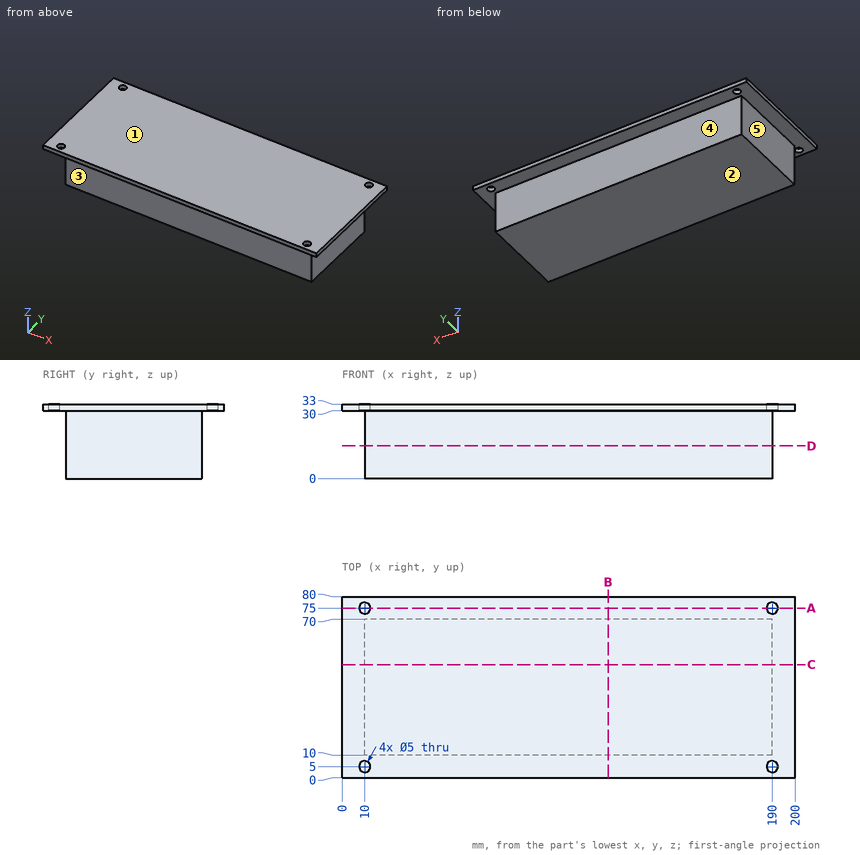
Could you check a few things on this drawing? It's one solid part, dimensions in mm from its lowest x, y, z. A direction names the side the tool comes from. Coordinates: 2 decimals unless noted, no trailing zeros. Order: outer loops, then holes, each group sorted by start corner. A loop starts at its lowest first (then second) coordinate and runs counter-clockwise, first axis right, second up. Notation, with made-up numbers: (11.25, 20.5) -> (56.25, 20.5) arc R17 cw to (56.25, 36.5) -> close; hole circle Ø2 at (-5.75, 52). An arc over 180 degrees is marked (long way). Answer in a Markdown table with one row per item.
(1) I want a section at D-D on z = 14.5. List the corners of the cut face in (x, y) for me, then the cut area to 3 significant figures.
Answer key:
| item | result |
|---|---|
| outline | (10, 10) -> (190, 10) -> (190, 70) -> (10, 70) -> close |
| area | 10,800 mm^2 |
(2) On a 3-axis mill with a long thin cutter (end or side, diameter ignored), from which of +Z, -Z, +X, -X, +Y, -Y can I reach the whole of each face in a straight line? I mean the marked faces 1, 2, 3, 4 and 5. Say none if no direction works.
Answer key:
| item | result |
|---|---|
| face 1 | +Z, +X, -X, +Y, -Y |
| face 2 | -Z, +X, -X, +Y, -Y |
| face 3 | -Z, +X, -X, -Y |
| face 4 | -Z, +X, -X, +Y |
| face 5 | -Z, -X, +Y, -Y |
(3) Will these pins go through, and if not, where does the flat tip stop? pin 1 Ø12 at (y, z) = (14, 22) entering from -X; pin 2 Ø6 at (y, z) = (66.5, 7.5) entering from +X; pin 3 Ø1.5 at (x, z) = (157.5, 23.5) entering from -Y.
Answer key:
| item | result |
|---|---|
| pin 1 | x = 10 |
| pin 2 | x = 190 |
| pin 3 | y = 10 |
(4) I want a section at A-A on y = 75. List the corners of the cut face in (x, z) for me, then the cut area to 3 significant figures.
Answer key:
| item | result |
|---|---|
| outline | (0, 30) -> (7.5, 30) -> (7.5, 33) -> (0, 33) -> close; (12.5, 30) -> (187.5, 30) -> (187.5, 33) -> (12.5, 33) -> close; (192.5, 30) -> (200, 30) -> (200, 33) -> (192.5, 33) -> close |
| area | 570 mm^2 |
(5) Please list where these lines run through material, in increasing order: probe 1 along Y at (x, z) = (10, 31); probe 2 along X at (y, z) = (28, 22); probe 3 along Y at (x, z) = (150, 16).
Answer key:
| item | result |
|---|---|
| probe 1 | 0 to 2.5, 7.5 to 72.5, 77.5 to 80 |
| probe 2 | 10 to 190 |
| probe 3 | 10 to 70 |
(6) I want a section at B-B on x = 117.5. List the corners of the cut face in (y, z) for me, then the cut area to 3 significant figures.
Answer key:
| item | result |
|---|---|
| outline | (0, 30) -> (10, 30) -> (10, 0) -> (70, 0) -> (70, 30) -> (80, 30) -> (80, 33) -> (0, 33) -> close |
| area | 2,040 mm^2 |
(7) I want a section at C-C on y = 50. List the corners of the cut face in (x, z) for me.
Answer key:
| item | result |
|---|---|
| outline | (0, 30) -> (10, 30) -> (10, 0) -> (190, 0) -> (190, 30) -> (200, 30) -> (200, 33) -> (0, 33) -> close |
